```python
from build123d import *

# Parameters (mm, degrees)
SKETCH2_R           = 17.25
BOSS_EXTRUDE1_DEPTH = 22.4
SKETCH3_R           = 14.9
BOSS_EXTRUDE2_DEPTH = 38.4
SKETCH4_R           = 14.9
BOSS_EXTRUDE3_DEPTH = 13.4
BOSS_EXTRUDE4_DEPTH = 14
SKETCH7_W           = 8
SKETCH7_H           = 12
BOSS_EXTRUDE5_DEPTH = 10
SKETCH9_W           = 3
SKETCH9_H           = 10
CUT_EXTRUDE1_DEPTH  = 2
SKETCH10_W          = 47.910910278
SKETCH10_H          = 37.599432614
BOSS_EXTRUDE6_DEPTH = 20
SKETCH12_R          = 6
CUT_EXTRUDE2_DEPTH  = 8


with BuildPart() as part:
    # Sketch2 → Boss-Extrude1 (new body)
    with BuildSketch(Plane.XY):
        Circle(SKETCH2_R)
    extrude(amount=BOSS_EXTRUDE1_DEPTH)

    # Sketch3 → Boss-Extrude2 (add)
    with BuildSketch(Plane.XY.offset(22.4)):
        Circle(SKETCH3_R)
    extrude(amount=BOSS_EXTRUDE2_DEPTH)

    # Sketch4 → Boss-Extrude3 (add)
    with BuildSketch(Plane.XY.offset(60.8)):
        Circle(SKETCH4_R)
    extrude(amount=BOSS_EXTRUDE3_DEPTH)

    # Sketch6 → Boss-Extrude4 (add)
    with BuildSketch(Plane.XY.offset(74.2)):
        with BuildLine():
            Line((0, 14.9), (23.472492354, 14.9))
            ThreePointArc((23.472492354, 14.9), (38.372492354, 0), (23.472492354, -14.9))
            Line((23.472492354, -14.9), (0, -14.9))
            ThreePointArc((0, -14.9), (-14.9, 0), (0, 14.9))
        make_face()
    extrude(amount=BOSS_EXTRUDE4_DEPTH)

    # Sketch7 → Boss-Extrude5 (add)
    with BuildSketch(Plane(origin=(0, 0, 0), x_dir=(-1, 0, 0), z_dir=(0, 0, -1))):
        Rectangle(SKETCH7_W, SKETCH7_H)
    extrude(amount=BOSS_EXTRUDE5_DEPTH)

    # Sketch9 → Cut-Extrude1 (cut)
    with BuildSketch(Plane(origin=(0, 0, -10), x_dir=(-1, 0, 0), z_dir=(0, 0, -1))):
        Rectangle(SKETCH9_W, SKETCH9_H)
    extrude(amount=-CUT_EXTRUDE1_DEPTH, mode=Mode.SUBTRACT)

    # Sketch10 → Boss-Extrude6 (add)
    with BuildSketch(Plane(origin=(0, 0, 0), x_dir=(-1, 0, 0), z_dir=(0, 0, -1))):
        Rectangle(SKETCH10_W, SKETCH10_H)
    extrude(amount=-BOSS_EXTRUDE6_DEPTH)

    # Sketch12 → Cut-Extrude2 (cut)
    with BuildSketch(Plane.XZ.offset(18.799716307)):
        with Locations(Location((0, 10, 0), (0, 0, 270))):
            Circle(SKETCH12_R)
    cut_extrude2 = extrude(amount=-CUT_EXTRUDE2_DEPTH, mode=Mode.SUBTRACT)

    # Mirror1: Cut-Extrude2 across plane
    add(cut_extrude2.mirror(Plane(origin=(0, 0, 0), x_dir=(0, 0, 1), z_dir=(0, -1, 0))), mode=Mode.SUBTRACT)


solid = part.part
```
Can you work these out from the model? Positions are in its coordinate system, mm. A direction names the side the tool comes from. Coordinates: 2 decimals unless noted, no trailing zeros. Loops run counter-clockwise (first coordinate to the right, second up) from the corner with the lowest first, then second, coordinate; pieces in that order, holes last. Notation, with made-up numbers: M -16,56.25 L -9,56.25 A27 cw -9,76.25 Z; hole C 13.5,59.25 d9. An arc over 180 degrees is marked long. Put each result on its own line as item: value. Start each with the question number.
(1) We'd pull the mould along Z, two halves only. Please class faces 1 (the face through (6, 17, 20)), 2 (the face through (12, 0, 88.2)), 3 (the face through (12, 14.9, 81)): +Z half, -Z half, draft (parallel to the pull), parting line (faces both ways), or undercut.
(2) Imagine slicing it at C-C on x = 16. List the corners of the cut face in (y, z) for me, and give its area (3 significant figures).
(3) Imagine slicing it at D-D on x = -9. List the corners of the cut face in (y, z) for me, and give its area (3 significant figures).
(4) Will these pins go through, and if not, where does the flat tip stop? pin 1 Ø10 at (y, z) = (1.5, 10.5) entering from +X; pin 2 Ø5 at (y, z) = (-2.5, -6) entering from +X; pin 3 Ø4 at (x, z) = (13.5, 39.5) entering from +Y; pin 4 Ø13 at (x, z) = (1.5, 9) entering from +Y.
(5) Which directions (+Z, -Z, +X, -X, +Y, -Y) give clear straight access to the entire face, cutting with the end or side of a thin tool? Please do faces 4 (the face through (0, -6, -5)), 5 (the face through (23.955, 0, 10)), 6 (the face through (16.453, 5.181, 21.183)).
(6) Imagine slicing it at B-B on y = 0. List the corners of the cut face in (x, z) for me.
(7) Imagine slicing it at A-A on z = 10. List the corners of the cut face in (x, y) for me, and give its area (3 significant figures).
(8) I need wall thicknesses on probe 1 along Z at (x, y) = (23, 1); probe 2 along X at (y, z) = (-14.75, 10); probe 3 along Z at (x, y) = (-5, -6). Which ranges of each line are inside material? Lowest first, please.
Worked answers:
1. face 1: undercut
1. face 2: +Z half
1. face 3: draft
2. outline: M -18.8,0 L 18.8,0 L 18.8,20 L 6.45,20 L 6.45,22.4 L -6.45,22.4 L -6.45,20 L -18.8,20 Z; M -14.9,74.2 L 14.9,74.2 L 14.9,88.2 L -14.9,88.2 Z
2. area: 1,200 mm2
3. outline: M -18.8,0 L 18.8,0 L 18.8,20 L 14.72,20 L 14.72,22.4 L 11.87,22.4 L 11.87,88.2 L -11.87,88.2 L -11.87,22.4 L -14.72,22.4 L -14.72,20 L -18.8,20 Z
3. area: 2,390 mm2
4. pin 1: stops at x = 23.96
4. pin 2: stops at x = 4
4. pin 3: stops at y = 9.47
4. pin 4: stops at y = 18.8
5. face 4: -Z, +X, -X, -Y
5. face 5: -Z, +X, +Y, -Y
5. face 6: none
6. outline: M -23.96,0 L -4,0 L -4,-10 L -1.5,-10 L -1.5,-8 L 1.5,-8 L 1.5,-10 L 4,-10 L 4,0 L 23.96,0 L 23.96,20 L 17.25,20 L 17.25,22.4 L 14.9,22.4 L 14.9,74.2 L 38.37,74.2 L 38.37,88.2 L -14.9,88.2 L -14.9,22.4 L -17.25,22.4 L -17.25,20 L -23.96,20 Z
7. outline: M -23.96,-18.8 L -6,-18.8 L -6,-10.8 L 6,-10.8 L 6,-18.8 L 23.96,-18.8 L 23.96,18.8 L 6,18.8 L 6,10.8 L -6,10.8 L -6,18.8 L -23.96,18.8 Z
7. area: 1,610 mm2
8. probe 1: z = 0 to 20, 74.2 to 88.2
8. probe 2: x = -23.96 to -6, 6 to 23.96
8. probe 3: z = 0 to 88.2
